Source: CAD feature listing. Evaluate the final solid. Frame: model axes, mm. A direction names the side the tool comes from. Round coordinates to 2 decimals unless told otherwise and drop trailing zeros. Loops run counter-clockwise (first coordinate to the right, second up) from the corner with the lowest first, then second, coordinate; pieces in that order, holes last. Notation, with made-up numbers: (-15.75, 54.5) -> (38.25, 54.5) arc R12 ccw to (38.25, 72.5) -> close; hole circle Ø6 at (-26.75, 1.5). An arc over 180 degrees is marked (long way). Write item = value, one per line.
Autodesk Inventor part; units mm, degrees
ref_plane "YZ Plane" through (0, 0, 0) normal (1, 0, 0) x (0, 1, 0)
ref_plane "XZ Plane" through (0, 0, 0) normal (0, 1, 0) x (-1, 0, 0)
ref_plane "XY Plane" through (0, 0, 0) normal (0, 0, 1) x (1, 0, 0)
sketch "_____1" plane through (0, 0, 0) normal (1, 0, 0) x (0, 0, -1)
  arc A0 (-35, 1) -> (-34, 0) centre (-34, 1) ccw
  line L0 (-34, 0) -> (-0.3, 0)
  arc A1 (-0.3, 0) -> (0, 0.3) centre (-0.3, 0.3) ccw
  line L1 (0, 0.3) -> (0, 34)
  arc A2 (0, 34) -> (-1, 35) centre (-1, 34) ccw
  line L2 (-1, 35) -> (-4, 35)
  arc A3 (-4, 35) -> (-5, 34) centre (-4, 34) ccw
  line L3 (-5, 34) -> (-5, 17.1243)
  arc A4 (-5.0879, 16.9121) -> (-5, 17.1243) centre (-5.3, 17.1243) ccw
  line L4 (-5.0879, 16.9121) -> (-7.6986, 14.3014)
  arc A5 (-8.1663, 14.3564) -> (-7.6986, 14.3014) centre (-7.9107, 14.5135) ccw
  arc A6 (-8.1663, 14.3564) -> (-14.3564, 8.1663) centre (-12, 12) ccw
  arc A7 (-14.3014, 7.6986) -> (-14.3564, 8.1663) centre (-14.5135, 7.9107) ccw
  line L5 (-14.3014, 7.6986) -> (-16.9121, 5.0879)
  arc A8 (-17.1243, 5) -> (-16.9121, 5.0879) centre (-17.1243, 5.3) ccw
  line L6 (-17.1243, 5) -> (-34, 5)
  arc A9 (-34, 5) -> (-35, 4) centre (-34, 4) ccw
  line L7 (-35, 4) -> (-35, 1)
extrude "Extrusion1" add sketch "_____1" along normal mid plane 9
sketch "_____2" plane through (0, 0, 0) normal (1, 0, 0) x (0, 0, -1)
  line L0 (-16.8296, 13.2941) -> (-13.9801, 12.5306)
  arc A0 (-13.9801, 12.5306) -> (-12.5306, 13.9801) centre (-12, 12) ccw
  line L1 (-12.5306, 13.9801) -> (-13.2941, 16.8296)
  arc A1 (-13.2941, 16.8296) -> (-16.8296, 13.2941) centre (-12, 12) ccw
extrude "Extrusion2" cut sketch "_____2" along normal mid plane 9
sketch "Sketch3" plane through (4.5, 34, 0) normal (0, 0, -1) x (-1, 0, 0)
  point P0 (4.5, -9)
hole "Hole1" at (0, 25, 0) direction (0, 0, 1) diameter 3.4 depth 5
sketch "Sketch4" plane through (-4.5, 5, 34) normal (0, 1, 0) x (1, 0, 0)
  point P0 (4.5, 9)
hole "Hole2" at (0, 5, 25) direction (0, -1, 0) diameter 3.4 depth 5
properties part number "HBLTBS3"
1. Line query: probe 1 along X at (y, z) = (25, 2.4); probe 2 along Y at (x, z) = (0, 1.5). Output: solid intervals per line, ascending. Write a range as from..to.
Evaluation:
probe_1 = -4.5..-1.7, 1.7..4.5
probe_2 = 0..23.3, 26.7..35
2. Contact query for flat-ended pins moving along their axis: pin 1 Ø4.5 at (x, z) = (0, 25) entering from +Y; pin 2 Ø2.5 at (x, y) = (0.5, 23) entering from +Z; pin 3 Ø1.5 at (x, z) = (2.5, 17) entering from +Y. Output: stop coordinate, or through.
Evaluation:
pin_1 = 5
pin_2 = 5
pin_3 = 13.16
3. Section query A-A (x = 0). Give the number of separate pieces and of enclosed holes in the cut face, then the cut area to 3 significant figures.
Evaluation:
separate_pieces = 3
enclosed_holes = 0
area = 385 mm²
4. Section query B-B (y = 25). Return the cut outline in (x, z).
Evaluation:
outline = (-4.5, 0) -> (-1.7, 0) -> (-1.7, 5) -> (-4.5, 5) -> close; (1.7, 0) -> (4.5, 0) -> (4.5, 5) -> (1.7, 5) -> close
5. Section query D-D (y = 3.5). Return the cut outline in (x, z).
Evaluation:
outline = (-4.5, 0) -> (4.5, 0) -> (4.5, 35) -> (-4.5, 35) -> close; hole circle Ø3.4 at (0, 25)
6. Section query C-C (z = 12). Return the cut outline in (x, y), then the cut area to 3 significant figures.
Evaluation:
outline = (-4.5, 0) -> (4.5, 0) -> (4.5, 9.95) -> (-4.5, 9.95) -> close; (-4.5, 14.05) -> (4.5, 14.05) -> (4.5, 16.5) -> (-4.5, 16.5) -> close
area = 112 mm²
7. Mould query, pull axis X, two halves, no side actions, for faces 1 (the face through (0.65, 2.46, 26.57)), 2 (the face through (0, 0, 17)), 3 (the face through (-4.5, 10, 11)). Classes: released by +X, released by -X, zero draft, split by the parting line, or undercut.
Evaluation:
face_1 = undercut
face_2 = zero draft
face_3 = released by -X
8. Set-up query: faces 4 (the face through (0, 28, 5)), 5 (the face through (-0.063, 15.147, 12.843)), 6 (the face through (-0.063, 12.852, 15.18)), 7 (the face through (-0.063, 0.285, 34.699)), 8 (the face through (0.65, 26.57, 2.54)). Return all of +Z, -Z, +X, -X, +Y, -Y with unobstructed straight access to the full face (end or side cutting, diameter ignored); none if empty.
Evaluation:
face_4 = +Z, +X, -X, +Y
face_5 = +Z, +X, -X
face_6 = +X, -X, +Y
face_7 = +Z, +X, -X, -Y
face_8 = +Z, -Z
